```python
from build123d import *

# Parameters (mm, degrees)
F0_R     = 1.25
F1_DEPTH = 3


with BuildPart() as f1:
    # F0 (on Front) → F1 (new body)
    with BuildSketch(Plane.XZ):
        with BuildLine():
            ThreePointArc((-10, -1), (-11, 0), (-10, 1))
            Line((-10, 1), (-4.898979, 1))
            ThreePointArc((-4.898979, 1), (-3.634068, 0.549193), (-2.939388, -0.6))
            ThreePointArc((-2.939388, -0.6), (2.32379, -1.897367), (0, 3))
            Line((0, 3), (-10, 3))
            ThreePointArc((-10, 3), (-13, 0), (-10, -3))
            Line((-10, -3), (-10, -1))
        make_face()
        Circle(F0_R, mode=Mode.SUBTRACT)
        with BuildLine():
            Line((-9.224745, -1), (-10, -1))
            Line((-10, -1), (-10, -3))
            Line((-10, -3), (-8, -3))
            ThreePointArc((-8, -3), (-6.842725, -1.277544), (-8.874818, -0.857143))
            ThreePointArc((-8.874818, -0.857143), (-9.035763, -0.96291), (-9.224745, -1))
        make_face()
    extrude(amount=F1_DEPTH)


solid = f1.part
```
Could you check a few things on this model? Use its own coordinates, in mm. A direction names the side the tool comes from. Coordinates: 2 decimals unless noted, no trailing zeros. Write each loop counter-clockwise with the first axis right and the second up, starting at its lowest first coordinate (ties: lowest second). Pieces come first, ordered by that corner, then holes. Notation, with made-up numbers: (-22, 87.5) -> (5, 87.5) arc R15 ccw to (5, 93.5) -> close; hole circle Ø3 at (18.25, -12). An arc over 180 degrees is marked (long way). Return JSON: item names as keys, results as strings.
(1) Imagine slicing it at A-A, the plane y = -0.2. Please give me the cut outline in (x, z).
Numbers:
{"outline": "(-10, -3) -> (-8, -3) arc R1.25 ccw (long way) to (-8.87, -0.86) arc R0.5 cw to (-9.22, -1) -> (-10, -1) arc R1 cw to (-10, 1) -> (-4.9, 1) arc R2 cw to (-2.94, -0.6) arc R3 ccw (long way) to (0, 3) -> (-10, 3) arc R3 ccw to start; hole circle Ø2.5 at (0, 0)"}
(2) Imagine slicing it at C-C, the plane z = 0. Please give me the cut outline in (x, y), then the cut area to 3 significant figures.
Numbers:
{"outline": "(-13, -3) -> (-11, -3) -> (-11, 0) -> (-13, 0) -> close; (-3.17, -3) -> (-1.25, -3) -> (-1.25, 0) -> (-3.17, 0) -> close; (1.25, -3) -> (3, -3) -> (3, 0) -> (1.25, 0) -> close", "area": "17.0 mm2"}
(3) Imagine slicing it at B-B, the plane x = -7.75. Please give me the cut outline in (y, z).
Numbers:
{"outline": "(-3, -2.97) -> (0, -2.97) -> (0, -0.53) -> (-3, -0.53) -> close; (-3, 1) -> (0, 1) -> (0, 3) -> (-3, 3) -> close"}
(4) Which directions (+Z, -Z, +X, -X, +Y, -Y) give clear straight access to the entire face, cutting with the end or side of a thin tool? Please do faces 1 (the flat face through (-5.1, -3, 1.4)), 2 (the cylindrical face through (-11, -1, 0)), 3 (the cylindrical face through (-3.65, -1.48, 0.56)).
Numbers:
{"face 1": "+Z, -Z, +X, -X, -Y", "face 2": "+Y, -Y", "face 3": "-Z, +Y, -Y"}
(5) Imagine slicing it at D-D, the plane x = -5.5. Please give me the cut outline in (y, z).
Numbers:
{"outline": "(-3, 1) -> (0, 1) -> (0, 3) -> (-3, 3) -> close"}
(6) We'd pull the mould along X, two halves only. Please class faces 4 (the cylindrical face through (-7, -1, -1)), 5 (the flat face through (-7, -1, 1)), 6 (the flat face through (-9, -1, -3)), 7 (the cylindrical face through (-13, -1, 0)): +X half, -X half, draft (parallel to the pull), parting line (faces both ways), or undercut.
Numbers:
{"face 4": "undercut", "face 5": "undercut", "face 6": "draft", "face 7": "-X half"}
(7) I need wall thicknesses on L1, parallel to Z at x = 0, y = -2.4; L2, parallel to Z at x = -10, y = -0.7; L3, parallel to X at y = -1.55, z = -1.5. Which ranges of each line are inside material? Lowest first, please.
Numbers:
{"L1": "z = -3 to -1.25, 1.25 to 3", "L2": "z = -3 to -1, 1 to 3", "L3": "x = -12.6 to -6.78, -2.6 to 2.6"}
